Here's how the part is built. I have some questions about the finished solid (model axes, mm). Face numbers are marked on the shaded views. Round coordinates to 2 decimals unless told otherwise and drop trailing zeros. Order: outer loops, then holes, each group sorted by start corner. A loop starts at its lowest first (then second) coordinate and runs counter-clockwise, first axis right, second up. Notation, with made-up numbers: M 87.25,65 L 93.25,65 A26 cw 93.25,97 Z; hole C -39,42 d7. An arc over 180 degrees is marked long. Use one line per item in the form item = value. Start each with the question number.
```python
from build123d import *

# Parameters (mm, degrees)
SKETCH1_R               = 3
SKETCH1_R_2             = 1.75
BOSS_EXTRUDE1_DEPTH     = 5
SKETCH3_W               = 8
SKETCH3_H               = 3
SKETCH3_H_2             = 4.010495491
SKETCH4_R               = 1.5
CUT_EXTRUDE1_DEPTH      = 10
CUT_EXTRUDE3_DEPTH      = 72.508687789
CUT_EXTRUDE3_DEPTH_BACK = 72.508687789
SKETCH7_W               = 18
SKETCH7_H               = 5
FILLET2_R               = 2
FILLET3_R               = 0.5


with BuildPart() as part:
    # Sketch1 → Boss-Extrude1 (new, symmetric)
    with BuildSketch(Plane(origin=(0, 0, 0), x_dir=(1, 0, 0), z_dir=(0, 1, 0))):
        with BuildLine():
            Line((-15.965575011, 4), (-9.729992932, 3.92576688))
            ThreePointArc((-9.729992932, 3.92576688), (27.429895786, 0.455123348), (64.661875809, 3.040149395))
            Line((64.661875809, 3.040149395), (68.034424989, 3))
            ThreePointArc((68.034424989, 3), (71.034424989, 0), (68.034424989, -3))
            Line((68.034424989, -3), (64.661875809, -3.040149395))
            ThreePointArc((64.661875809, -3.040149395), (27.50198709, -6.510792927), (-9.729992932, -3.92576688))
            Line((-9.729992932, -3.92576688), (-15.965575011, -4))
            ThreePointArc((-15.965575011, -4), (-19.965575011, 0), (-15.965575011, 4))
        make_face()
        with Locations(Location((-15.965575011, 0, 0), (0, 0, 270))):
            Circle(SKETCH1_R, mode=Mode.SUBTRACT)
        with Locations(Location((68.034424989, 0, 0), (0, 0, 270))):
            Circle(SKETCH1_R_2, mode=Mode.SUBTRACT)
    extrude(amount=BOSS_EXTRUDE1_DEPTH, both=True)

    # Sketch3 → Cut-Revolve1 (revolve, cut)
    with BuildSketch(Plane(origin=(68.034424989, 0, 0), x_dir=(0, 0, -1), z_dir=(1, 0, 0))):
        with Locations((4, -3.5)):
            Rectangle(SKETCH3_W, SKETCH3_H)
        with Locations((4, 4.005247746)):
            Rectangle(SKETCH3_W, SKETCH3_H_2)
    revolve(axis=Axis((68.034424989, 6.010495491, 0), (0, -1, 0)), mode=Mode.SUBTRACT)

    # Sketch4 → Cut-Extrude1 (cut)
    with BuildSketch(Plane(origin=(0, 5, 0), x_dir=(1, 0, 0), z_dir=(0, 1, 0))):
        with Locations(Location((32.466788231, -3.022809684, 0), (0, 0, 270))):
            Circle(SKETCH4_R)
    extrude(amount=-CUT_EXTRUDE1_DEPTH, mode=Mode.SUBTRACT)

    # Sketch7 → Cut-Extrude3 (cut, two sides: drawn at the far end of the back side and taken through both)
    with BuildSketch(Plane.XY.offset(-CUT_EXTRUDE3_DEPTH_BACK)):
        with Locations((32.466788231, -2.5)):
            Rectangle(SKETCH7_W, SKETCH7_H)
    extrude(amount=CUT_EXTRUDE3_DEPTH + CUT_EXTRUDE3_DEPTH_BACK, mode=Mode.SUBTRACT)

    # Fillet2
    fillet2_edges = [part.edges().sort_by_distance(p)[0] for p in [
        (23.466788231, -2.5, 6.523430697),
        (23.466788231, -2.5, -0.536463963),
        (41.466788231, -2.5, 5.919808824),
        (41.466788231, -2.5, -0.716531943),
    ]]
    fillet(fillet2_edges, radius=FILLET2_R)

    # Fillet3
    # the kernel refuses this fillet: 0.5 mm, written as the material it adds along each edge
    with BuildSketch(Plane(origin=(23.466788231, 0, 1.397952858), x_dir=(0, -1, 0), z_dir=(0, 0, 1))) as fillet3_piece_1:
        with BuildLine():
            CenterArc((FILLET3_R, FILLET3_R), FILLET3_R, 180, 90)
            Line((0, FILLET3_R), (0, 0))
            Line((0, 0), (FILLET3_R, 0))
        make_face()
    extrude(amount=3.105292794)
    with BuildSketch(Plane(origin=(41.466788231, 0, 3.758708932), x_dir=(0, -1, 0), z_dir=(0, 0, -1))) as fillet3_piece_2:
        with BuildLine():
            CenterArc((FILLET3_R, FILLET3_R), FILLET3_R, 180, 90)
            Line((0, FILLET3_R), (0, 0))
            Line((0, 0), (FILLET3_R, 0))
        make_face()
    extrude(amount=2.579020088)
    with BuildSketch(Plane(origin=(21.466788231, 0, 1.397952858), x_dir=(1, 0, 0), z_dir=(0, 0, 1))) as fillet3_piece_3_section:
        with BuildLine():
            CenterArc((2 + FILLET3_R, -FILLET3_R), FILLET3_R, 90, 90)
            Line((2 + FILLET3_R, 0), (2, 0))
            Line((2, 0), (2, -FILLET3_R))
        make_face()
    fillet3_piece_3 = revolve(axis=Axis((21.466788231, 0, 1.397952858), (0, 1, 0)), revolution_arc=123.674223315, mode=Mode.PRIVATE)
    fillet3_piece_3 = fillet3_piece_3 - Plane(origin=(30.167797019, -0.143096894, -230.438826894), x_dir=(-0.17346865196054342, 0, 0.9848393913664257), z_dir=(0, 1, 0)) * Cylinder(230, 10, mode=Mode.PRIVATE)
    add(fillet3_piece_3)
    with BuildSketch(Plane(origin=(43.466788231, 0, 1.179688844), x_dir=(-1, 0, 0), z_dir=(0, 0, 1))) as fillet3_piece_4_section:
        with BuildLine():
            CenterArc((2 + FILLET3_R, FILLET3_R), FILLET3_R, 180, 90)
            Line((2 + FILLET3_R, 0), (2, 0))
            Line((2, 0), (2, FILLET3_R))
        make_face()
    fillet3_piece_4 = revolve(axis=Axis((43.466788231, 0, 1.179688844), (0, -1, 0)), revolution_arc=122.537034738, mode=Mode.PRIVATE)
    fillet3_piece_4 = fillet3_piece_4 - Plane(origin=(30.167797019, -0.143120672, -230.438826894), x_dir=(-0.17346865196054342, 0, 0.9848393913664257), z_dir=(0, 1, 0)) * Cylinder(230, 10, mode=Mode.PRIVATE)
    add(fillet3_piece_4)
    with BuildSketch(Plane(origin=(43.466788231, 0, 3.758708932), x_dir=(0.6498595886550582, 0, 0.7600542842673006), z_dir=(0.7600542842673006, 0, -0.6498595886550582))) as fillet3_piece_5_section:
        with BuildLine():
            CenterArc((2 + FILLET3_R, FILLET3_R), FILLET3_R, 180, 90)
            Line((2, FILLET3_R), (2, 0))
            Line((2, 0), (2 + FILLET3_R, 0))
        make_face()
    fillet3_piece_5 = revolve(axis=Axis((43.466788231, 0, 3.758708932), (0, -1, 0)), revolution_arc=130.531016297, mode=Mode.PRIVATE)
    fillet3_piece_5 = fillet3_piece_5 & Plane(origin=(24.764085858, -0.142965197, -223.472910619), x_dir=(0.1734686519605446, 0, 0.9848393913664256), z_dir=(0, 1, 0)) * Cylinder(230, 11, mode=Mode.PRIVATE)
    add(fillet3_piece_5)
    with BuildSketch(Plane(origin=(21.466788231, 0, 4.503245652), x_dir=(-0.5969692661029794, 0, 0.8022641057210962), z_dir=(-0.8022641057210962, 0, -0.5969692661029794))) as fillet3_piece_6_section:
        with BuildLine():
            CenterArc((2 + FILLET3_R, -FILLET3_R), FILLET3_R, 90, 90)
            Line((2 + FILLET3_R, 0), (2, 0))
            Line((2, 0), (2, -FILLET3_R))
        make_face()
    fillet3_piece_6 = revolve(axis=Axis((21.466788231, 0, 4.503245652), (0, 1, 0)), revolution_arc=126.653144299, mode=Mode.PRIVATE)
    fillet3_piece_6 = fillet3_piece_6 & Plane(origin=(24.764085858, -0.14303929, -223.472910619), x_dir=(0.1734686519605446, 0, 0.9848393913664256), z_dir=(0, 1, 0)) * Cylinder(230, 11, mode=Mode.PRIVATE)
    add(fillet3_piece_6)


solid = part.part
```
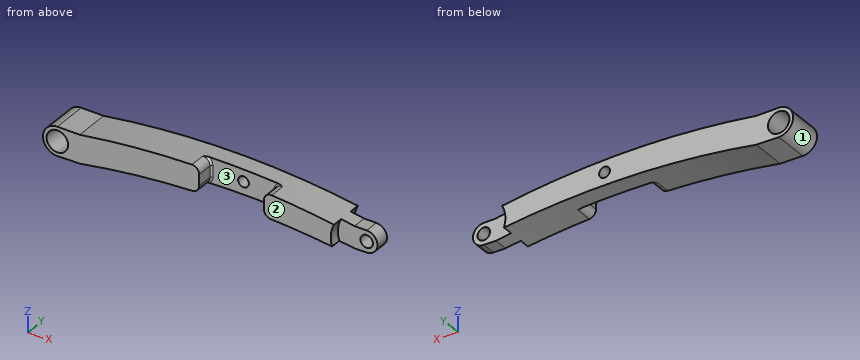
1) If I drill on line 1 (X direction, y = 0.5, z = 0); line 2 (X direction, y = 1, z = 1); line 3 (X direction, y = -1.2, z = 0), over which ranges is the centre line in solid material (lowest first)?
2) If we section it at A-A on y = -3.5: Write out the boundary of the cut face in (x, z).
3) If we mould it in two halves opening along X, with no side actions, what happens to the marked faces 1, 2 and 3? For each: +X half, -X half, draft (parallel to the pull), parting line (faces both ways), or undercut.
4) If we section it at B-B on x = 58: Write out the boundary of the cut face in (y, z), then the cut area to 3 significant figures.
5) Will these pins go through, and if not, where does the flat tip stop? pin 1 Ø1 at (y, z) = (-1.5, 1) entering from +X; pin 2 Ø2 at (x, z) = (66.5, 0.5) entering from +Y; pin 3 Ø4 at (y, z) = (1.5, 3) entering from +X; pin 4 Ø1.8 at (x, z) = (32.47, 3.02) entering from +Y.
6) If we section it at C-C on x = 38: Write out the boundary of the cut face in (y, z), then the cut area to 3 significant figures.
Completed:
q1.line_1 = -19.97 to -18.97, -12.97 to 66.28, 69.78 to 71.03
q1.line_2 = -19.84 to -18.79, -13.14 to 66.6, 69.47 to 70.86
q1.line_3 = -19.97 to -18.97, -12.97 to 22.9, 41.85 to 66.28, 69.78 to 71.03
q2.outline = M -15.97,-4 L -9.73,-3.93 A230 cw 21.54,-0.6 A2 ccw 23.47,1.4 L 23.47,4.5 A2 ccw 21.44,6.5 A230 ccw -9.73,3.93 L -15.97,4 A4 ccw Z; M 41.47,1.18 A2 ccw 43.35,-0.82 A230 cw 60.41,-2.44 A8 cw 60.92,3.67 A230 ccw 43.63,5.75 A2 ccw 41.47,3.76 Z; hole C -15.97,0 d6
q3.face_1 = -X half
q3.face_2 = draft
q3.face_3 = undercut
q4.outline = M -5,-2.13 L 5,-2.13 L 5,4.11 L -5,4.11 Z
q4.area = 62.4 mm²
q5.pin_1 = 70.99
q5.pin_2 = 2
q5.pin_3 = 70.86
q5.pin_4 = through
q6.outline = M 0,-0.57 L 5,-0.57 L 5,6.15 L 0,6.15 Z
q6.area = 33.6 mm²
